Autodesk Inventor part; units mm, degrees
ref_plane "YZ Plane" through (0, 0, 0) normal (1, 0, 0) x (0, 1, 0)
ref_plane "XZ Plane" through (0, 0, 0) normal (0, 1, 0) x (-1, 0, 0)
ref_plane "XY Plane" through (0, 0, 0) normal (0, 0, 1) x (1, 0, 0)
sketch "Sketch1" plane through (0, 0, 0) normal (0, 0, 1) x (1, 0, 0)
  circle A0 centre (0, 0) radius 55
  circle A1 centre (0, 0) radius 14
  circle A2 centre (0, 0) radius 40 construction
  circle A3 centre (40, 0) radius 4
  circle A4 centre (28.2843, 28.2843) radius 4
  circle A5 centre (0, 40) radius 4
  circle A6 centre (-28.2843, 28.2843) radius 4
  circle A7 centre (-40, 0) radius 4
  circle A8 centre (-28.2843, -28.2843) radius 4
  circle A9 centre (0, -40) radius 4
  circle A10 centre (28.2843, -28.2843) radius 4
  dimension "d39" = 80
  dimension "d31" = 28
  dimension "d32" = 110
  dimension "d40" = 8
  dimension "d43" = 360
extrude "Plate1" add sketch "Sketch1" against normal blind 2
equation "\"d15\" = Thickness"
equation "\"BendRadius\" = Thickness"
equation "\"BendReliefWidth\" = Thickness"
equation "\"BendReliefDepth\" = 0.5 * Thickness"
equation "\"CornerReliefSize\" = 4 * Thickness"
equation "\"MinimumRemnant\" = 2 * Thickness"
equation "\"TransitionRadius\" = BendRadius"
equation "\"JacobiRadiusSize\" = BendRadius"
equation "\"GapSize\" = Thickness"
properties part number "flange small gear"
The listing builds one solid part. Answer for the finished solid, in the listing's coordinates (mm). Coordinates: 2 decimals unless noted, no trailing zeros. Write each loop counter-clockwise with the first axis right and the second up, starting at its lowest first coordinate (ties: lowest second). Pieces come first, ordered by that corner, then holes. Notation, with made-up numbers: M 57.5,-30.75 L 69.5,-30.75 A35 cw 69.5,6.25 Z; hole C 41.5,81 d4. An arc over 180 degrees is marked long. Use one line per item in the form item = value.
Item 1: Given P1, Ø5, axis at x = -28.28, y = 28.28, coming from the -Z side, flat-ended and moving along its own axis, determine where the tip first touches the part or whether it passes through.
Model answer:
P1 = through
Item 2: Find section C-C, the plane z = -0.4. Give the number of separate pieces and of enclosed holes in the cut face, plus the area to 3 significant figures.
Model answer:
separate_pieces = 1
enclosed_holes = 9
area = 8,490 mm2
Item 3: Find section A-A, the plane x = 0. Give the vertices of the cut face in (y, z).
Model answer:
outline = M -55,-2 L -44,-2 L -44,0 L -55,0 Z; M -36,-2 L -14,-2 L -14,0 L -36,0 Z; M 14,-2 L 36,-2 L 36,0 L 14,0 Z; M 44,-2 L 55,-2 L 55,0 L 44,0 Z
Item 4: Find the intervals of material crossed by probe 1 along Y at (x, z) = (0, -0.75); probe 2 along Y at (x, z) = (-27, -0.6), in increasing order.
Model answer:
probe_1 = -55 to -44, -36 to -14, 14 to 36, 44 to 55
probe_2 = -47.92 to -32.07, -24.5 to 24.5, 32.07 to 47.92
Item 5: The mould has two halves that part along Y. Classify faces 1 (the face through (11, -11, 0)), 2 (the face through (-0.521, -36.034, -0.986)), 3 (the face through (-11.923, -53.692, -0.986)): released by +Y, released by -Y, zero draft, split by the parting line, or undercut.
Model answer:
face_1 = zero draft
face_2 = undercut
face_3 = split by the parting line
Item 6: Find section D-D, the plane x = 41.5. Give the vertices of the cut face in (y, z).
Model answer:
outline = M -36.09,-2 L -3.71,-2 L -3.71,0 L -36.09,0 Z; M 3.71,-2 L 36.09,-2 L 36.09,0 L 3.71,0 Z
